Could you check a few things on this model? Use its own coordinates, in mm. A direction names the side the tool comes from. Give positions to 0.01 mm unless a question says otherwise; leave off trailing zeros. Loops run counter-clockwise (first coordinate to the right, second up) from the corner with the lowest first, then second, coordinate; pieces in that order, holes last. Notation, with made-up numbers: (70.25, 52.5) -> (88.25, 52.5) arc R14 ccw to (88.25, 79.5) -> close; hole circle Ø9 at (-28, 55.5). An arc over 180 degrees is marked (long way). Write each question's results on one line, items separated by ' | '. Start each with the question number.
Q1. If we section it at C-C, the plane z = 4: List the corners of the cut face in (x, y) for me.
Q2. Will these pins go through, and if not, where does the flat tip stop? P1, Ø10, axis at x = 6.5, z = 10, coming from the -Y side; P2, Ø2, axis at x = -21.5, z = 8.5, coming from the +Y side; P3, Ø1, axis at y = 3.5, z = 10.5, coming from the +X side.
Q3. If we section it at B-B, the plane x = 0: List the corners of the cut face in (y, z) for me, plus the area to 3 significant figures.
Q4. If we section it at A-A, the plane z = 10: List the corners of the cut face in (x, y) for me.
Q5. We'd pull the mould along X, two halves only. Please class faces 6 (the face through (-12.077, -2.851, 9.86)), 7 (the face through (-5, 1, 20)), 8 (the face through (-24.52, 4.66, 9.86)): released by +X, released by -X, zero draft, split by the parting line, or undercut.
Q6. If I drill on line 1 along X through (y, z) = (2, 11.25); line 2 along Z through (x, y) = (0, 1.5); line 3 along X through (y, z) = (3.25, 19), over which ranges is the centre line in solid material (lowest first)?
Q7. Which directions (+Z, -Z, +X, -X, +Y, -Y) give clear straight access to the entire face, cutting with the end or side of a thin tool? Please do faces 1 (the face through (-2.4, 2.5, 7.6)), 2 (the face through (-2.4, -2.5, 7.6)), 3 (the face through (-16.382, -2.897, 9.86)), 4 (the face through (-21.313, 0.521, 9.86)), 5 (the face through (-22.14, 2.34, 9.86)).
Q8. If we section it at D-D, the plane x = -5: List the corners of the cut face in (y, z) for me, plus the area to 3 significant figures.
from build123d import *

# Parameters (mm, degrees)
F0_W      = 20
F0_H      = 5
F1_DEPTH  = 20
F2_R      = 2.75
F3_DEPTH  = 6.3
F3_FACE_R = 2.75
F4_DEPTH  = 6.5967602214
F5_R      = 2


# Not quite as in the source:
# - a feature names something its author has since deleted; it is built from what else it names


with BuildPart() as f1:
    # F0 (on Top) → F1 (new body)
    with BuildSketch(Plane.XY):
        Polygon((-10, -2.5), (-10, 2.5), (-17.9419796384, 8.0610340111), (-23.1064327086, 6.6772229816), (-21.8777046422, 5.8168583271), (-11.2287280664, -1.6396353455), align=None)
        Rectangle(F0_W, F0_H)
        Polygon((-21.8777046422, 5.8168583271), (-23.1064327086, 6.6772229816), (-25.9743148904, 2.5814627602), (-21.8785546689, -0.2864194216), (-20.7314017962, 1.351884667), (-23.5984339512, 3.3594021942), align=None)
        Polygon((-12.8678821818, -6.5957602214), (-10, -2.5), (-11.2287280664, -1.6396353455), (-12.9494573755, -4.0970914783), (-15.8164895305, -2.0895739511), (-16.9636424032, -3.7278780397), align=None)
    extrude(amount=F1_DEPTH)

    # F2 (on Front) → F3 (cut)
    with BuildSketch(Plane.XZ):
        with Locations((0, 10)):
            Circle(F2_R)
    extrude(amount=-F3_DEPTH, mode=Mode.SUBTRACT)

    # F2 (on Front) + F3_face (on face) → F4 (cut, through all)
    with BuildSketch(Plane.XZ):
        with Locations((0, 10)):
            Circle(F2_R)
    with BuildSketch(Plane(origin=(0, 0, 10), x_dir=(-1, 0, 0), z_dir=(0, 1, 0))):
        Circle(F3_FACE_R)
    extrude(amount=F4_DEPTH, dir=(0, -1, 0), mode=Mode.SUBTRACT)

    # F5
    f5_edges = [f1.edges().sort_by_distance(p)[0] for p in [
        (10, 0, 20),
        (10, 0, 0),
    ]]
    fillet(f5_edges, radius=F5_R)


solid = f1.part
Final values:
1) outline: (-25.97, 2.58) -> (-21.88, -0.29) -> (-20.73, 1.35) -> (-23.6, 3.36) -> (-21.88, 5.82) -> (-11.23, -1.64) -> (-12.95, -4.1) -> (-15.82, -2.09) -> (-16.96, -3.73) -> (-12.87, -6.6) -> (-10, -2.5) -> (10, -2.5) -> (10, 2.5) -> (-10, 2.5) -> (-17.94, 8.06) -> (-23.11, 6.68) -> close
2) P1: stops at y = -2.5 | P2: stops at y = 7.38 | P3: stops at x = -10.71
3) outline: (-2.5, 0) -> (2.5, 0) -> (2.5, 7.25) -> (-2.5, 7.25) -> close; (-2.5, 12.75) -> (2.5, 12.75) -> (2.5, 20) -> (-2.5, 20) -> close | area: 72.5 mm²
4) outline: (-25.97, 2.58) -> (-21.88, -0.29) -> (-20.73, 1.35) -> (-23.6, 3.36) -> (-21.88, 5.82) -> (-11.23, -1.64) -> (-12.95, -4.1) -> (-15.82, -2.09) -> (-16.96, -3.73) -> (-12.87, -6.6) -> (-10, -2.5) -> (-2.75, -2.5) -> (-2.75, 2.5) -> (-10, 2.5) -> (-17.94, 8.06) -> (-23.11, 6.68) -> close; (2.75, -2.5) -> (10, -2.5) -> (10, 2.5) -> (2.75, 2.5) -> close
5) face 6: undercut | face 7: zero draft | face 8: released by -X
6) line 1: x = -25.14 to -21.66, -16.43 to -2.45, 2.45 to 10 | line 2: z = 0 to 7.25, 12.75 to 20 | line 3: x = -25.51 to -23.44, -18.21 to -11.07
7) face 1: +Z, -Z, +X, +Y | face 2: +Z, -Z, +X, -Y | face 3: +Z, -Z, -X | face 4: +Z, -Z, -Y | face 5: +Z, -Z
8) outline: (-2.5, 0) -> (2.5, 0) -> (2.5, 20) -> (-2.5, 20) -> close | area: 100 mm²
